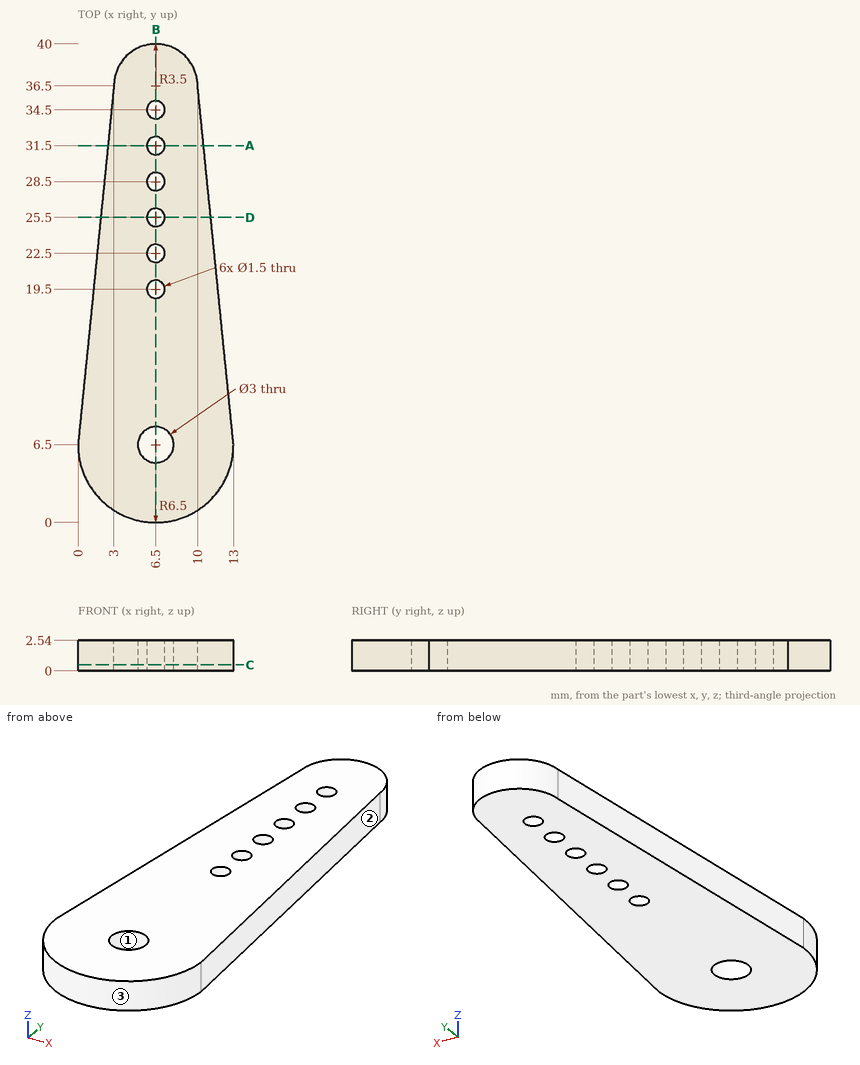
Input: dimensioned drawing with shaded views. Units: mm. Origin: part minimum x, y, z. Coordinates: 2 decimals unless noted, no trailing zeros. Loops run counter-clockwise (first coordinate to the right, second up) from the corner with the lowest first, then second, coordinate; pieces in that order, holes last. Notation, with made-up numbers: M 87.5,64.25 L 118.5,64.25 A30 ccw 118.5,89.25 Z; hole C -35,67 d9. An arc over 180 degrees is marked long. Put each result on its own line as item: value.
(1) First-contact query: pin 1 (1 mm diameter, centred on y = 20.5, z = 2, fed in from +X). Flat tip, straight axial feed; report the tip coordinate or a pass-through.
Answer sheet:
pin 1: stops at x = 11.65
(2) Cut plane C-C on z = 0.5. Return the cut outline in (x, y), then the cut area to 3 significant figures.
Answer sheet:
outline: M 0,6.5 A6.5 ccw 13,6.5 L 10,36.5 A3.5 ccw 3,36.5 Z; hole C 6.5,6.5 d3; hole C 6.5,19.5 d1.5; hole C 6.5,22.5 d1.5; hole C 6.5,25.5 d1.5; hole C 6.5,28.5 d1.5; hole C 6.5,31.5 d1.5; hole C 6.5,34.5 d1.5
area: 368 mm^2
(3) Cut plane A-A on y = 31.5. Return the cut outline in (x, z), then the cut area to 3 significant figures.
Answer sheet:
outline: M 2.5,0 L 5.75,0 L 5.75,2.54 L 2.5,2.54 Z; M 7.25,0 L 10.5,0 L 10.5,2.54 L 7.25,2.54 Z
area: 16.5 mm^2
(4) Cut plane D-D on y = 25.5. Return the cut outline in (x, z).
Answer sheet:
outline: M 1.9,0 L 5.75,0 L 5.75,2.54 L 1.9,2.54 Z; M 7.25,0 L 11.1,0 L 11.1,2.54 L 7.25,2.54 Z
(5) Draft query along Y for the marked faces 1, 2 and 3. Return one class per face: pulls with the +Y half, pulls with the -Y half, needs draft (parallel to the pull), parting line crosses it, or undercut.
Answer sheet:
face 1: undercut
face 2: pulls with the +Y half
face 3: pulls with the -Y half
(6) Material intervals for probe 1 along X at (y, z) = (19.5, 1.95); probe 2 along X at (y, z) = (34.5, 0.9); probe 3 along X at (y, z) = (27.5, 0.3), sorted ascending.
Answer sheet:
probe 1: x = 1.3 to 5.75, 7.25 to 11.7
probe 2: x = 2.8 to 5.75, 7.25 to 10.2
probe 3: x = 2.1 to 10.9
(7) Cut plane B-B on x = 6.5. State how many separate pieces and enclosed holes the cut face has, then the cut area to 3 significant figures.
Answer sheet:
separate pieces: 8
enclosed holes: 0
area: 71.1 mm^2
